CAD build for the part. Positions are in the model's coordinates, mm. A direction names the side the tool comes from. Round coordinates to 2 decimals unless told otherwise and drop trailing zeros. Write each loop counter-clockwise with the first axis right and the second up, starting at its lowest first coordinate (ties: lowest second). Pieces come first, ordered by that corner, then holes. Notation, with made-up numbers: (85, 73.25) - (117, 73.25) arc R23 cw to (117, 102.25) - close; hole circle Ø8 at (59, 11.25). An arc over 180 degrees is marked (long way). Put each result on its own line as item: value. Start each with the question number.
Item 1: Cut at A-A (y = 1.75). Give the cut face in (x, z) (3 decimals), and give its area (3 significant figures).
Item 2: Cut at D-D (z = -10.5). Give the cut face in (x, y) (3 decimals).
Item 3: 3-axis set-ups, long thin cutter, end or side, ignore diameter. For faces 4 (the flat face through (6, 0, -6)), 5 (the flat face through (0.635, 1, -6)): which of +Z, -Z, +X, -X, +Y, -Y reach the whole face in a straight line?
Item 4: Cut at C-C (x = 1). Give the cut face in (y, z) (3 decimals), and give its area (3 significant figures).
Item 5: Drill centre lines: line 1 (Z direction, x = 3.5, y = 0.3) (3 decimals); line 2 (X direction, y = 0.7, z = -11.5) (3 decimals); line 3 (X direction, y = 1.85, z = -8.5) (3 decimals). Where is each one in solid material? Low to high. Write a range as from..to.
Item 6: Mould opens along Z. For faces 1 (the cylindrical face through (8.83, 0.97, -6.9)), 2 (the flat face through (0, 1, -6)), 3 (the flat face through (6, 1, -12.7)) say: released by +Z, released by -Z, zero draft, split by the parting line, or undercut.
```python
from build123d import *

# Parameters (mm, degrees)
SKETCH1_W           = 12.7
SKETCH1_H           = 12.7
BOSS_EXTRUDE1_DEPTH = 2.54
FILLET1_R           = 0.635
SHELL1_START        = 0.635
SHELL1_OUTLINE_W    = 1.905
SHELL1_OUTLINE_H    = 11.43
SHELL1_DEPTH        = 11.43
SKETCH2_R           = 2.54
BOSS_EXTRUDE2_DEPTH = 1.905
BOSS_EXTRUDE3_DEPTH = 0.00254


# Read off the part's stored shape, not the designer's step: Shell1
with BuildPart() as part:
    # Sketch1 → Boss-Extrude1 (new body)
    with BuildSketch(Plane(origin=(0, 0, 0), x_dir=(1, 0, 0), z_dir=(0, 1, 0))):
        with Locations((6.35, 6.35)):
            Rectangle(SKETCH1_W, SKETCH1_H)
    extrude(amount=BOSS_EXTRUDE1_DEPTH)

    # Fillet1
    fillet1_edges = [part.edges().sort_by_distance(p)[0] for p in [
        (0, 1.27, -12.7),
        (12.7, 1.27, -12.7),
        (12.7, 1.27, 0),
        (0, 1.27, 0),
    ]]
    fillet(fillet1_edges, radius=FILLET1_R)

    # Shell1 outline → Shell1 (cut)
    with BuildSketch(Plane.YZ.offset(SHELL1_START)):
        with Locations((0.9525, -6.35)):
            Rectangle(SHELL1_OUTLINE_W, SHELL1_OUTLINE_H)
    extrude(amount=SHELL1_DEPTH, mode=Mode.SUBTRACT)

    # Sketch2 → Boss-Extrude2 (add)
    with BuildSketch(Plane(origin=(0, 1.905, 0), x_dir=(-1, 0, 0), z_dir=(0, -1, 0))):
        with Locations(Location((-6.35, 6.35, 0), (0, 0, 270))):
            Circle(SKETCH2_R)
    extrude(amount=BOSS_EXTRUDE2_DEPTH)

    # Sketch3 → Boss-Extrude3 (add)
    with BuildSketch(Plane(origin=(0, 2.54, 0), x_dir=(1, 0, 0), z_dir=(0, 1, 0))):
        Polygon((5.497146154, 8.001), (6.067017949, 8.001), (6.067017949, 5.395871795), (6.962530769, 5.395871795), (6.962530769, 4.826), (5.497146154, 4.826), align=None)
    extrude(amount=BOSS_EXTRUDE3_DEPTH)


solid = part.part
```
Output values:
1. outline: (0, -12.065) arc R0.635 ccw to (0.635, -12.7) - (12.065, -12.7) arc R0.635 ccw to (12.7, -12.065) - (12.7, -0.635) arc R0.635 ccw to (12.065, 0) - (0.635, 0) arc R0.635 ccw to (0, -0.635) - close; circle Ø5.08 at (6.35, -6.35); hole (0.635, -12.065) - (12.065, -12.065) - (12.065, -0.635) - (0.635, -0.635) - close
1. area: 50.6 mm2
2. outline: (0, 0) - (0.635, 0) - (0.635, 1.905) - (12.065, 1.905) - (12.065, 0) - (12.7, 0) - (12.7, 2.54) - (0, 2.54) - close
3. face 4: +Z, -Z, +X, -X, -Y
3. face 5: -Y
4. outline: (0, -12.7) - (2.54, -12.7) - (2.54, 0) - (0, 0) - (0, -0.635) - (1.905, -0.635) - (1.905, -12.065) - (0, -12.065) - close
4. area: 10.5 mm2
5. line 1: -12.7..-12.065, -0.635..0
5. line 2: 0..0.635, 12.065..12.7
5. line 3: 0..0.635, 4.998..7.702, 12.065..12.7
6. face 1: undercut
6. face 2: zero draft
6. face 3: released by -Z
